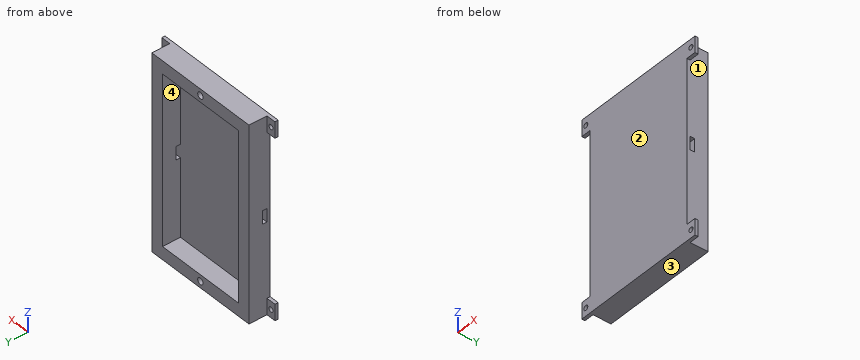
from build123d import *

# Parameters (mm, degrees)
ESBO_O1_W                = 36.4
ESBO_O1_H                = 60.4
ESBO_O1_W_2              = 28.4
ESBO_O1_H_2              = 52.4
RESSALTO_EXTRUS_O1_DEPTH = 6.6
ESBO_O2_W                = 28.4
ESBO_O2_H                = 52.4
RESSALTO_EXTRUS_O2_DEPTH = 1
ESBO_O4_W                = 4.1
ESBO_O4_H                = 1.4
CORTE_EXTRUS_O2_DEPTH    = 38
ESBO_O5_W                = 3
ESBO_O5_H                = 5
ESBO_O5_R                = 0.75
RESSALTO_EXTRUS_O3_DEPTH = 1
ESBO_O6_R                = 1
CORTE_EXTRUS_O3_DEPTH    = 4


with BuildPart() as part:
    # Esboço1 → Ressalto-extrusão1 (new body)
    with BuildSketch(Plane(origin=(0, 0, 0), x_dir=(1, 0, 0), z_dir=(0, 1, 0))):
        Rectangle(ESBO_O1_W, ESBO_O1_H)
        Rectangle(ESBO_O1_W_2, ESBO_O1_H_2, mode=Mode.SUBTRACT)
    extrude(amount=RESSALTO_EXTRUS_O1_DEPTH)

    # Esboço2 → Ressalto-extrusão2 (add)
    with BuildSketch(Plane(origin=(0, 0, 0), x_dir=(1, 0, 0), z_dir=(0, 1, 0))):
        Rectangle(ESBO_O2_W, ESBO_O2_H)
    extrude(amount=RESSALTO_EXTRUS_O2_DEPTH)

    # Esboço4 → Corte-extrusão2 (cut)
    with BuildSketch(Plane(origin=(18.2, 0, 0), x_dir=(0, 0, -1), z_dir=(1, 0, 0))):
        with Locations((0, 1.7)):
            Rectangle(ESBO_O4_W, ESBO_O4_H)
    extrude(amount=-CORTE_EXTRUS_O2_DEPTH, mode=Mode.SUBTRACT)

    # Esboço5 → Ressalto-extrusão3 (add)
    # profile 1 of 4: a face of its own
    with BuildSketch(Plane(origin=(0, 0, 0), x_dir=(1, 0, 0), z_dir=(0, 1, 0))):
        with Locations((-19.7, 27.7)):
            Rectangle(ESBO_O5_W, ESBO_O5_H)
        with Locations(Location((-19.7, 27.7, 0), (0, 0, 270))):
            Circle(ESBO_O5_R, mode=Mode.SUBTRACT)
    # profile 2 of 4: a face of its own
    with BuildSketch(Plane(origin=(0, 0, 0), x_dir=(1, 0, 0), z_dir=(0, 1, 0))):
        with Locations((-19.7, -27.7)):
            Rectangle(ESBO_O5_W, ESBO_O5_H)
        with Locations(Location((-19.7, -27.7, 0), (0, 0, 270))):
            Circle(ESBO_O5_R, mode=Mode.SUBTRACT)
    # profile 3 of 4: a face of its own
    with BuildSketch(Plane(origin=(0, 0, 0), x_dir=(1, 0, 0), z_dir=(0, 1, 0))):
        with Locations((19.7, -27.7)):
            Rectangle(ESBO_O5_W, ESBO_O5_H)
        with Locations(Location((19.7, -27.7, 0), (0, 0, 270))):
            Circle(ESBO_O5_R, mode=Mode.SUBTRACT)
    # profile 4 of 4: a face of its own
    with BuildSketch(Plane(origin=(0, 0, 0), x_dir=(1, 0, 0), z_dir=(0, 1, 0))):
        with Locations((19.7, 27.7)):
            Rectangle(ESBO_O5_W, ESBO_O5_H)
        with Locations(Location((19.7, 27.7, 0), (0, 0, 270))):
            Circle(ESBO_O5_R, mode=Mode.SUBTRACT)
    extrude(amount=RESSALTO_EXTRUS_O3_DEPTH)

    # Esboço6 → Corte-extrusão3 (cut)
    with BuildSketch(Plane(origin=(0, 6.6, 0), x_dir=(1, 0, 0), z_dir=(0, 1, 0))):
        with Locations(Location((0, 28.2, 0), (0, 0, 270))):
            Circle(ESBO_O6_R)
        with Locations(Location((0, -28.2, 0), (0, 0, 270))):
            Circle(ESBO_O6_R)
    extrude(amount=-CORTE_EXTRUS_O3_DEPTH, mode=Mode.SUBTRACT)


solid = part.part
Part model, mm, in its own coordinate system. Face numbers are marked on the shaded views. A direction names the side the tool comes from. Coordinates: 2 decimals unless noted, no trailing zeros. Write each loop counter-clockwise with the first axis right and the second up, starting at its lowest first coordinate (ties: lowest second). Pieces come first, ordered by that corner, then holes. Notation, with made-up numbers: M 79.25,-9.75 L 132.25,-9.75 A12 cw 132.25,7.25 Z; hole C 66,7 d1. An arc over 180 degrees is marked long. Return JSON: item names as keys, results as strings.
1. Saw through at C-C, the plane z = -4.5. Write the cut outline in (x, y).
Determined:
{"outline": "M -18.2,0 L 18.2,0 L 18.2,6.6 L 14.2,6.6 L 14.2,1 L -14.2,1 L -14.2,6.6 L -18.2,6.6 Z"}
2. Pull direction Y, two halves, no side cores. Call the marked faces 1 and 2: pulls with the +Y half, pulls with the -Y half, needs draft (parallel to the pull), parting line crosses it, or undercut.
Determined:
{"face 1": "needs draft", "face 2": "pulls with the -Y half"}
3. Probe L1, parallel to X at y = 0.7, z = 27.7; L2, parallel to Z at x = -18, y = 1.25; L3, parallel to Z at x = -9, y = 4. List the from-to ranges inside material, lowest first.
Determined:
{"L1": "-21.2 to -20.45, -18.95 to 18.95, 20.45 to 21.2", "L2": "-30.2 to -2.05, 2.05 to 30.2", "L3": "-30.2 to -26.2, 26.2 to 30.2"}
4. Saw through at B-B, the plane y = 3.75. Write the cut outline in (x, z).
Determined:
{"outline": "M -18.2,-30.2 L 18.2,-30.2 L 18.2,30.2 L -18.2,30.2 Z; hole M -14.2,-26.2 L 14.2,-26.2 L 14.2,26.2 L -14.2,26.2 Z; hole C 0,-28.2 d2; hole C 0,28.2 d2"}
5. Flat gauge pins, fed straight in: pin 1 Ø1.5 at (y, z) = (2, -17.5) entering from +X; pin 2 Ø1.2 at (x, z) = (-19.7, 27.7) entering from -Y; pin 3 Ø2 at (y, z) = (2, -14.5) entering from -X; pin 4 Ø18 at (x, z) = (-1.5, 6.5) entering from +Y. Where does each tip first touch, or does it go through?
Determined:
{"pin 1": "x = 18.2", "pin 2": "through", "pin 3": "x = -18.2", "pin 4": "y = 1"}
6. Saw through at A-A, the plane x = 19.7. Write the cut outline in (y, z), then the cut area to 3 significant figures.
Determined:
{"outline": "M 0,-30.2 L 1,-30.2 L 1,-28.45 L 0,-28.45 Z; M 0,-26.95 L 1,-26.95 L 1,-25.2 L 0,-25.2 Z; M 0,25.2 L 1,25.2 L 1,26.95 L 0,26.95 Z; M 0,28.45 L 1,28.45 L 1,30.2 L 0,30.2 Z", "area": "7.00 mm²"}
7. 3-axis set-ups, long thin cutter, end or side, ignore diameter. For the marked faces 3 and 4: which of +Z, -Z, +X, -X, +Y, -Y reach the whole face in a straight line?
Determined:
{"face 3": "-Z, +X, -X, +Y, -Y", "face 4": "+Y"}
8. Saw through at D-D, the plane x = 10.5. Write the cut outline in (y, z), then the cut area to 3 significant figures.
Determined:
{"outline": "M 0,-30.2 L 6.6,-30.2 L 6.6,-26.2 L 1,-26.2 L 1,26.2 L 6.6,26.2 L 6.6,30.2 L 0,30.2 Z", "area": "105 mm²"}
